Autodesk Fusion 360 part; units mm, degrees
sketch "Sketch1" plane through (0, 0, 0) normal (0, 0, 1) x (1, 0, 0)
  line L0 (0, 0) -> (56, 0)
  line L1 (56, 0) -> (56, 105)
  line L2 (56, 105) -> (0, 105)
  line L3 (0, 105) -> (0, 0)
  dimension "d1" = 56
  dimension "d2" = 105
extrude "Extrude1" add sketch "Sketch1" along normal blind 5
sketch "Sketch2" plane through (0, 0, 5) normal (0, 0, 1) x (-1, 0, 0)
  line L0 (0, -105) -> (0, 0)
  line L1 (0, 0) -> (-56, 0)
  line L2 (-56, 0) -> (-56, -105)
  line L3 (-56, -105) -> (0, -105)
  circle A0 centre (-3.5, -91) radius 1.35
  circle A1 centre (-52.5, -91) radius 1.35
  circle A2 centre (-3.5, -33) radius 1.35
  circle A3 centre (-52.5, -33) radius 1.35
  circle A4 centre (-3.5, -91) radius 3.5
  circle A5 centre (-52.5, -91) radius 3.5
  circle A6 centre (-52.5, -33) radius 3.5
  circle A7 centre (-3.5, -33) radius 3.5
  line L4 (-3.5, -36.5) -> (0, -36.5)
  line L5 (-3.5, -29.5) -> (0, -29.5)
  line L6 (-52.5, -29.5) -> (-56, -29.5)
  line L7 (-52.5, -87.5) -> (-56, -87.5)
  line L8 (-52.5, -94.5) -> (-56, -94.5)
  line L9 (-3.5, -94.5) -> (0, -94.5)
  line L10 (-3.5, -87.5) -> (0, -87.5)
  line L11 (-52.5, -36.5) -> (-56, -36.5)
  dimension "d5" = 2.7
  dimension "d6" = 58
  dimension "d7" = 49
  dimension "d8" = 3.5
  dimension "d9" = 56
  dimension "d10" = 105
  dimension "d11" = 33
extrude "Extrude2" add sketch "Sketch2" along normal blind 4 contours L0 A4 L9 | L0 A4 L10 | A4 | L2 A5 L8 | L2 A5 L7 | A5 | L0 A7 L4 | L0 A7 L5 | A7 | L2 A6 L11 | L2 A6 L6 | A6
extrude "Extrude3" cut sketch "Sketch2" against normal blind 7 contours A0 | A1 | A2 | A3
sketch "Sketch3" plane through (0, 0, 5) normal (0, 0, 1) x (-1, 0, 0)
  line L0 (-3.5, -29.5) -> (0, -29.5)
  line L1 (0, -29.5) -> (0, 0)
  line L2 (0, 0) -> (-56, 0)
  line L3 (-56, 0) -> (-56, -29.5)
  line L4 (-56, -29.5) -> (-52.5, -29.5)
  arc A0 (-52.5, -36.5) -> (-52.5, -29.5) centre (-52.5, -33) ccw
  line L5 (-52.5, -36.5) -> (-56, -36.5)
  line L6 (-56, -36.5) -> (-56, -87.5)
  line L7 (-56, -87.5) -> (-52.5, -87.5)
  arc A1 (-52.5, -94.5) -> (-52.5, -87.5) centre (-52.5, -91) ccw
  line L8 (-52.5, -94.5) -> (-56, -94.5)
  line L9 (-56, -94.5) -> (-56, -105)
  line L10 (-56, -105) -> (0, -105)
  line L11 (0, -105) -> (0, -94.5)
  line L12 (0, -94.5) -> (-3.5, -94.5)
  arc A2 (-3.5, -87.5) -> (-3.5, -94.5) centre (-3.5, -91) ccw
  line L13 (-3.5, -87.5) -> (0, -87.5)
  line L14 (0, -87.5) -> (0, -36.5)
  line L15 (0, -36.5) -> (-3.5, -36.5)
  arc A3 (-3.5, -29.5) -> (-3.5, -36.5) centre (-3.5, -33) ccw
  circle A4 centre (-5, -5) radius 1.5
  circle A5 centre (-51, -5) radius 1.5
  circle A6 centre (-51, -100) radius 1.5
  circle A7 centre (-5, -100) radius 1.5
  dimension "d16" = 5
  dimension "d17" = 5
  dimension "d18" = 5
  dimension "d19" = 3
  dimension "d20" = 5
extrude "Extrude4" cut sketch "Sketch3" against normal blind 5 contours A4 | A5 | A6 | A7
chamfer "Chamfer1" distance 1 distance2 1 4 edges at (6.3985, 4.4576, 5) (52.3985, 4.4576, 5) (52.3985, 99.4576, 5) (6.3985, 99.4576, 5) measured on face at (35.3731, 53.1886, 5) measured on face at (35.3731, 53.1886, 5) measured on face at (35.3731, 53.1886, 5) measured on face at (35.3731, 53.1886, 5)
sketch "Sketch4" plane through (0, 0, 0) normal (0, 0, -1) x (1, 0, 0)
  circle A0 centre (51, -100) radius 1.5
  circle A1 centre (5, -5) radius 1.5
  circle A2 centre (5, -100) radius 1.5
  circle A3 centre (51, -5) radius 1.5
  circle A4 centre (3.5, -91) radius 1.35
  circle A5 centre (52.5, -91) radius 1.35
  circle A6 centre (3.5, -33) radius 1.35
  circle A7 centre (52.5, -33) radius 1.35
  line L0 (0, 0) -> (0, -105)
  line L1 (0, -105) -> (56, -105)
  line L2 (56, -105) -> (56, 0)
  line L3 (56, 0) -> (0, 0)
  circle A8 centre (3.5, -91) radius 2
  circle A9 centre (52.5, -91) radius 2
  circle A10 centre (52.5, -33) radius 2
  circle A11 centre (3.5, -33) radius 2
  dimension "d25" = 4
extrude "Extrude5" cut sketch "Sketch4" against normal blind 5 contours A8 | A9 | A10 | A11
equation "d2 = 85 mm + 20 mm"
equation "d8 = ( d9 - d7 ) / 2"
equation "d11 = 23 mm + 10 mm"
equation "d17 = d16"
equation "d18 = d16"
The listing builds one solid part. Answer for the finished solid, in the listing's coordinates (mm). A direction names the side the tool comes from. Give positions to 0.01 mm unless a question says otherwise; leave off trailing zeros. Write each loop counter-clockwise with the first axis right and the second up, starting at its lowest first coordinate (ties: lowest second). Pieces come first, ordered by that corner, then holes. Notation, with made-up numbers: (-3.5, -29) -> (51.5, -29) arc R15 ccw to (51.5, -7) -> close; hole circle Ø3 at (33, 53). An arc over 180 degrees is marked (long way). One line per question, with ' | ' between items. Start each with the question number.
1. For faces 1 (the flat face through (54, 29.5, 7)), 2 (the flat face through (54, 87.5, 7)), 3 (the cylindrical face through (7, 33, 7)), 4 (the cylindrical face through (3.79, 31.68, 6.97)), 5 (the cylindrical face through (3.066, 34.952, 2.465)), determine the directions among +Z, -Z, +X, -X, +Y, -Y from which every point of the face is accessible in a straight line to the end or side of a thin tool.
2. Given pin 1 Ø1.8 at (x, z) = (54, 6.5) entering from -Y; pin 2 Ø8 at (x, y) = (6.5, 49.5) entering from +Z; pin 3 Ø1.8 at (x, z) = (54, 7) entering from +Y, each flat-ended and moving along its own axis, determine where each tip first touches the part or whether it passes through.
3. Section C-C (y = 33) is taken. Determine the outline of the cut face in (x, z), plus the area to 3 significant figures.
4. Section D-D (x = 39.5) is taken. Determine the outline of the cut face in (y, z).
5. Section A-A (z = 6) is taken. Determine the outline of the cut face in (x, y), plus the area to 3 significant figures.
6. Section B-B (y = 100) is taken. Determine the outline of the cut face in (x, z), plus the area to 3 significant figures.
7. For a pull along Y with two mould halves and no side action, classify faces 6 (the flat face through (54.1, 33, 9)), 7 (the flat face through (2, 94.5, 7)), 8 (the flat face through (5, 33, 5)), 9 (the flat face through (28, 0, 2)) as pulls with the +Y half, pulls with the -Y half, needs draft (parallel to the pull), parting line crosses it, or undercut.
8. Find the intervals of material crossed by probe 1 along X at (y, z) = (91, 7.35); probe 2 along X at (y, z) = (5, 1.75); probe 3 along Y at (x, z) = (52.5, 7.9), in increasing order.
Response values:
1) face 1: +Z, +X, -X, -Y | face 2: +Z, +X, -X | face 3: +Z | face 4: +Z, -Z | face 5: -Z
2) pin 1: y = 29.5 | pin 2: z = 5 | pin 3: y = 94.5
3) outline: (0, 0) -> (1.5, 0) -> (1.5, 5) -> (2.15, 5) -> (2.15, 9) -> (0, 9) -> close; (4.85, 5) -> (5.5, 5) -> (5.5, 0) -> (50.5, 0) -> (50.5, 5) -> (51.15, 5) -> (51.15, 9) -> (49, 9) -> (49, 5) -> (7, 5) -> (7, 9) -> (4.85, 9) -> close; (53.85, 5) -> (54.5, 5) -> (54.5, 0) -> (56, 0) -> (56, 9) -> (53.85, 9) -> close | area: 274 mm2
4) outline: (0, 0) -> (105, 0) -> (105, 5) -> (0, 5) -> close
5) outline: (0, 29.5) -> (3.5, 29.5) arc R3.5 ccw to (3.5, 36.5) -> (0, 36.5) -> close; (0, 87.5) -> (3.5, 87.5) arc R3.5 ccw to (3.5, 94.5) -> (0, 94.5) -> close; (52.5, 29.5) -> (56, 29.5) -> (56, 36.5) -> (52.5, 36.5) arc R3.5 ccw to start; (52.5, 87.5) -> (56, 87.5) -> (56, 94.5) -> (52.5, 94.5) arc R3.5 ccw to start; hole circle Ø2.7 at (3.5, 33); hole circle Ø2.7 at (3.5, 91); hole circle Ø2.7 at (52.5, 33); hole circle Ø2.7 at (52.5, 91) | area: 152 mm2
6) outline: (0, 0) -> (3.5, 0) -> (3.5, 4) -> (2.5, 5) -> (0, 5) -> close; (6.5, 0) -> (49.5, 0) -> (49.5, 4) -> (48.5, 5) -> (7.5, 5) -> (6.5, 4) -> close; (52.5, 0) -> (56, 0) -> (56, 5) -> (53.5, 5) -> (52.5, 4) -> close | area: 248 mm2
7) face 6: needs draft | face 7: pulls with the +Y half | face 8: undercut | face 9: pulls with the -Y half
8) probe 1: 0 to 2.15, 4.85 to 7, 49 to 51.15, 53.85 to 56 | probe 2: 0 to 3.5, 6.5 to 49.5, 52.5 to 56 | probe 3: 29.5 to 31.65, 34.35 to 36.5, 87.5 to 89.65, 92.35 to 94.5
